CAD build for the part. Positions are in the model's coordinates, mm. Round coordinates to 2 decimals unless told otherwise and drop trailing zeros. Order: outer loops, then holes, each group sorted by start corner. A loop starts at its lowest first (then second) coordinate and runs counter-clockwise, first axis right, second up. Notation, with made-up numbers: M -30.5,48.25 L -15.5,48.25 A23 ccw -15.5,59.25 Z; hole C -23.5,67.25 d2. An arc over 180 degrees is marked long. Put each result on its own line as item: value.
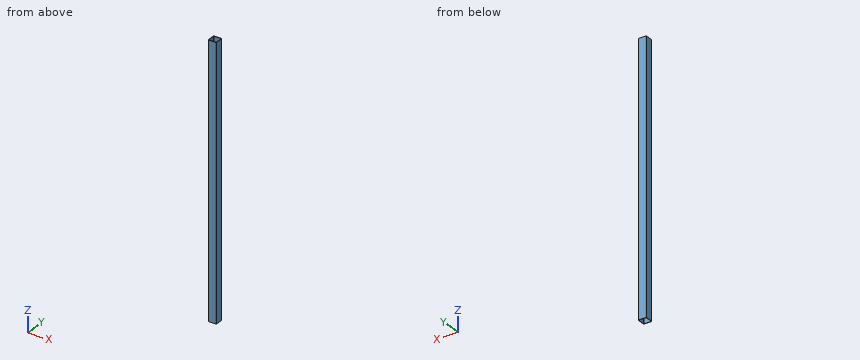
Autodesk Inventor part; units mm, degrees
ref_plane "Plano inicial" through (0, 0, 35) normal (0, 0, 1) x (1, 0, 0)
ref_plane "Plano final" through (0, 0, 2280) normal (0, 0, 1) x (1, 0, 0)
ref_plane "Plano de trabajo4" through (500, 29, 2280) normal (0, 0, 1) x (1, 0, 0)
ref_plane "Plano inicial" through (0, 0, 35) normal (0, 0, 1) x (1, 0, 0)
ref_plane "Plano final" through (0, 0, 2280) normal (0, 0, 1) x (1, 0, 0)
sketch "Boceto" plane through (0, 0, 0) normal (0, 0, 1) x (1, 0, 0)
  line L0 (-35, -29) -> (-35, 29)
  line L1 (-29, 35) -> (29, 35)
  line L2 (35, 29) -> (35, -29)
  line L3 (29, -35) -> (-29, -35)
  arc A0 (-35, -29) -> (-29, -35) centre (-29, -29) ccw
  arc A1 (35, 29) -> (29, 35) centre (29, 29) ccw
  arc A2 (-29, 35) -> (-35, 29) centre (-29, 29) ccw
  arc A3 (29, -35) -> (35, -29) centre (29, -29) ccw
  arc A4 (-29, 32) -> (-32, 29) centre (-29, 29) ccw
  line L4 (-29, 32) -> (29, 32)
  arc A5 (32, 29) -> (29, 32) centre (29, 29) ccw
  line L5 (32, 29) -> (32, -29)
  arc A6 (29, -32) -> (32, -29) centre (29, -29) ccw
  line L6 (29, -32) -> (-29, -32)
  arc A7 (-32, -29) -> (-29, -32) centre (-29, -29) ccw
  line L7 (-32, -29) -> (-32, 29)
  line L8 (0, 50.7397) -> (0, -50.7397) construction
  line L9 (-50.7397, 0) -> (50.7397, 0) construction
  dimension "d7" = 6
  dimension "d9" = 70
  dimension "d11" = 70
  dimension "d12" = 3
  dimension "d15" = 35
  dimension "d16" = 35
extrude "Cuerpo" add sketch "Boceto" along normal up to surface (2245 mm away) from surface at 35
sketch "Sketch3" plane through (0, 0, 0) normal (0, 0, 1) x (1, 0, 0)
  line L0 (0, 0) -> (10, 0)
ref_plane "Work Plane3" through (0, 0, 0) normal (0, -1, 0) x (1, 0, 0)
sketch "Sketch4" plane through (0, 0, 0) normal (0, -1, 0) x (1, 0, 0)
  line L0 (-2, 35) -> (12, 35)
  line L1 (-2, 2280) -> (12, 2280)
  dimension "d18" = 2245
ref_plane "Plano de trabajo4" through (500, 29, 2280) normal (0, 0, 1) x (1, 0, 0)
split "Dividir1" plane through (500, 29, 2280) removes the side toward (0, 0, 1)
ref_plane "Plano de trabajo5" through (1000, 29, 35) normal (0, 0, -1) x (-1, 0, 0)
split "Dividir2" plane through (1000, 29, 35) removes the side toward (0, 0, -1)
equation "\"d7\" = G_IR"
equation "\"d9\" = G_W"
equation "\"d11\" = G_H"
equation "\"d12\" = G_T"
equation "\"d15\" = 0.5 * d9"
equation "\"d16\" = 0.5 * d11"
equation "\"d3\" = G_L"
equation "\"G_W\" = 70"
equation "\"G_H\" = 70"
equation "\"G_T\" = 3"
equation "\"G_IR\" = 6"
equation "\"G_L\" = d18"
equation "\"G_OFFSET_START\" = -35"
equation "\"G_OFFSET_END\" = -35"
equation "\"d13\" = -G_OFFSET_START"
equation "\"B_L\" = 2315"
properties part number "ISO 10799-2 - 70x70x3 - 2245" material "Galvanizado catalogo 2"
Item 1: Band-saw the part on A-A on x = 6. Give the cut face in (y, z), and give its area (3 significant figures).
Answers below:
outline: M -35,35 L -32,35 L -32,2280 L -35,2280 Z; M 32,35 L 35,35 L 35,2280 L 32,2280 Z
area: 13,500 mm²
Item 2: Probe line 1 along Y through (x, z) = (6.5, 397); line 2 along Y through (x, z) = (30, 448). List the from-to ranges inside material, lowest first. Write a range as [from, to].
Answers below:
line 1: [-35, -32], [32, 35]
line 2: [-34.92, -31.83], [31.83, 34.92]
Item 3: Band-saw the part on B-B on z = 581. Give the cut face in (x, y), and give its area (3 significant figures).
Answers below:
outline: M -35,-29 A6 ccw -29,-35 L 29,-35 A6 ccw 35,-29 L 35,29 A6 ccw 29,35 L -29,35 A6 ccw -35,29 Z; hole M -32,-29 A3 ccw -29,-32 L 29,-32 A3 ccw 32,-29 L 32,29 A3 ccw 29,32 L -29,32 A3 ccw -32,29 Z
area: 781 mm²
